from build123d import *

# Parameters (mm, degrees)
ESQUISSE1_W             = 125
ESQUISSE1_H             = 130
BOSS_EXTRU_1_DEPTH      = 10
ENL_V_MAT_EXTRU_1_DEPTH = 125
ESQUISSE4_R             = 2.5
ENL_V_MAT_EXTRU_2_DEPTH = 3
CHANFREIN2_SIZE         = 2
ENL_V_MAT_EXTRU_6_DEPTH = 126


with BuildPart() as part:
    # Esquisse1 → Boss.-Extru.1 (new body)
    with BuildSketch(Plane(origin=(0, 0, 0), x_dir=(1, 0, 0), z_dir=(0, 1, 0))):
        with Locations((62.5, 65)):
            Rectangle(ESQUISSE1_W, ESQUISSE1_H)
    extrude(amount=BOSS_EXTRU_1_DEPTH)

    # Esquisse2 → Enlèv. mat.-Extru.1 (cut)
    with BuildSketch(Plane(origin=(125, 0, 0), x_dir=(0, 0, -1), z_dir=(1, 0, 0))):
        Polygon((8.2, 10), (8.2, 8.4), (3, 3.2), (3, 3), (23.6, 3), (23.6, 3.2), (18.4, 8.4), (18.4, 10), align=None)
        Polygon((118.6, 10), (118.6, 8.4), (123.8, 3.2), (123.8, 3), (103.2, 3), (103.2, 3.2), (108.4, 8.4), (108.4, 10), align=None)
    extrude(amount=-ENL_V_MAT_EXTRU_1_DEPTH, mode=Mode.SUBTRACT)

    # Esquisse4 → Enlèv. mat.-Extru.2 (cut)
    with BuildSketch(Plane(origin=(0, 3, 0), x_dir=(1, 0, 0), z_dir=(0, 1, 0))):
        with Locations((100, 13.3)):
            Circle(ESQUISSE4_R)
        with Locations((25, 13.3)):
            Circle(ESQUISSE4_R)
        with Locations((100, 113.5)):
            Circle(ESQUISSE4_R)
        with Locations((25, 113.5)):
            Circle(ESQUISSE4_R)
    extrude(amount=-ENL_V_MAT_EXTRU_2_DEPTH, mode=Mode.SUBTRACT)

    # Chanfrein2
    chanfrein2_edges = [part.edges().sort_by_distance(p)[0] for p in [
        (22.5, 3, -13.3),
        (97.5, 3, -113.5),
        (22.5, 3, -113.5),
        (97.5, 3, -13.3),
    ]]
    chamfer(chanfrein2_edges, length=CHANFREIN2_SIZE)

    # Esquisse8 → Enlèv. mat.-Extru.6 (cut, through all)
    with BuildSketch(Plane.ZY):
        Polygon((-105.4, 10), (-104.089482721, 8.689482721), (-98.479134235, 3.079134235), (-98.4, 3), (-28.4, 3), (-28.320865765, 3.079134235), (-22.710517279, 8.689482721), (-21.4, 10), align=None)
    extrude(amount=-ENL_V_MAT_EXTRU_6_DEPTH, mode=Mode.SUBTRACT)


solid = part.part
Geometry check sheet. Reference: the model listing, model coordinates, mm. A direction names the side the tool comes from. Coordinates: 2 decimals unless noted, no trailing zeros. Write each loop counter-clockwise with the first axis right and the second up, starting at its lowest first coordinate (ties: lowest second). Pieces come first, ordered by that corner, then holes. Notation, with made-up numbers: (28.25, -21.75) -> (68.25, -21.75) arc R19 cw to (68.25, -6.75) -> close; hole circle Ø9 at (50, 20). An arc over 180 degrees is marked (long way). One line per question, with ' | ' between items.
1. Cross-section at C-C on x = 25. State how many separate pieces and enclosed holes the cut face has, and give its area (3 significant figures).
Answers:
separate pieces: 3 | enclosed holes: 0 | area: 522 mm²
2. Draft check along Z on faces 4 (the flat face through (61.6, 6.5, -101.9)), 5 (the flat face through (62, 10, -4)), 6 (the flat face through (62, 5, 0)), 7 (the flat face through (62, 5, -130)). Enter one of: +Z half, -Z half, draft (parallel to the pull), parting line (faces both ways), or undercut.
Answers:
face 4: undercut | face 5: draft | face 6: +Z half | face 7: -Z half
3. Cross-section at A-A on z = -13.3. Record the cut outline in (x, y).
Answers:
outline: (0, 0) -> (22.5, 0) -> (22.5, 1) -> (20.5, 3) -> (0, 3) -> close; (27.5, 0) -> (97.5, 0) -> (97.5, 1) -> (95.5, 3) -> (29.5, 3) -> (27.5, 1) -> close; (102.5, 0) -> (125, 0) -> (125, 3) -> (104.5, 3) -> (102.5, 1) -> close
4. Depth check by flat-ended pin: pin 1 Ø6 at (y, z) = (5, -76) entering from -X; pin 2 Ø21 at (x, z) = (35, -49.5) entering from +Y; pin 3 Ø3 at (x, z) = (100, -113.5) entering from +Y. Enter the tip coordinate at first touch or a pass-through.
Answers:
pin 1: stops at x = 0 | pin 2: stops at y = 3 | pin 3: passes through
5. Thickness scan on probe 1 along X at (y, z) = (0.3, -13.3); probe 2 along Z at (x, y) = (100, 0.3); probe 3 along Z at (x, y) = (62.5, 7.5). Record the ranges inside material, lowest first. Write a range as from..to.
Answers:
probe 1: x = 0..22.5, 27.5..97.5, 102.5..125 | probe 2: z = -130..-116, -111..-15.8, -10.8..0 | probe 3: z = -130..-119.5, -107.5..-102.9, -23.9..-19.3, -7.3..0
6. Cross-section at B-B on x = 61. Record the cut outline in (y, z), and give its area (3 significant figures).
Answers:
outline: (0, -130) -> (10, -130) -> (10, -118.6) -> (8.4, -118.6) -> (3.2, -123.8) -> (3, -123.8) -> (3, -103.2) -> (3.2, -103.2) -> (8.4, -108.4) -> (10, -108.4) -> (10, -105.4) -> (3, -98.4) -> (3, -28.4) -> (10, -21.4) -> (10, -18.4) -> (8.4, -18.4) -> (3.2, -23.6) -> (3, -23.6) -> (3, -3) -> (3.2, -3) -> (8.4, -8.2) -> (10, -8.2) -> (10, 0) -> (0, 0) -> close | area: 560 mm²
7. Cross-section at D-D on z = -37.5. Record the cut outline in (x, y), and give its area (3 significant figures).
Answers:
outline: (0, 0) -> (125, 0) -> (125, 3) -> (0, 3) -> close | area: 375 mm²
8. Set-up check for faces 1 (the flat face through (63, 6, -121)), 2 (the cylindrical face through (102.385, 0.507, -14.051)), 3 (the flat face through (61.6, 6.5, -24.9)): record each of +Z, -Z, +X, -X, +Y, -Y from which the full face is reachable in a straight line by a thin tool's end or side.
Answers:
face 1: +X, -X | face 2: +Y, -Y | face 3: +X, -X, +Y
